Geometry: see drawing. Coordinates: mm, zero at the bounding-box minimum. A direction names the side the tool comes from. Coordinates: 2 decimals unless noted, no trailing zeros. Write each loop counter-clockwise with the first axis right and the second up, starting at its lowest first coordinate (ties: lowest second). Pieces come first, ordered by that corner, then holes. Notation, with made-up numbers: M 6,66.25 L 55,66.25 A17 ccw 55,84.25 Z; hole C 71,65.25 d10. An arc over 180 degrees is marked long. Answer as CSV lines item,"result". Start each with the question number.
1. Section C-C on x = 5. Return the cut outline in (y, z).
2. Section A-A on x = 14. Return the cut outline in (y, z), plus the area to 3 significant figures.
3. Contact query for flat-ended pins moving along their axis: pin 1 Ø5 at (y, z) = (6, 6.5) entering from -X; pin 2 Ø3.5 at (x, z) = (35, 18.5) entering from +Y; pin 3 Ø5.5 at (x, y) = (14.5, 9) entering from +Z; pin 4 Ø3.5 at (x, z) = (5, 18.5) entering from -Y. Output: stop coordinate, or through.
4. Section B-B on y = 3.5. Return the cut outline in (x, z).
5. Mould query, pull axis X, two halves, no side actions, for the marked faces 6, 7, 8 and 9. Classes: pulls with the +X half, pulls with the -X half, needs draft (parallel to the pull), parting line crosses it, or undercut.
6. Section D-D on y = 18. Return the cut outline in (x, z), plus the area to 3 significant figures.
7. Reachability of the marked faces 1, 2, 3, 4 and 5 from +Z, -Z, +X, -X, +Y, -Y: full face, straight path, thin tool, end or side. Return the list, or none.
8. Line query: probe 1 along Y at (x, z) = (14.1, 6.5); probe 2 along X at (y, z) = (14, 2.75); probe 3 along Y at (x, z) = (23, 5.5). Output: solid intervals per line, ascending. Write a range as [from, to].
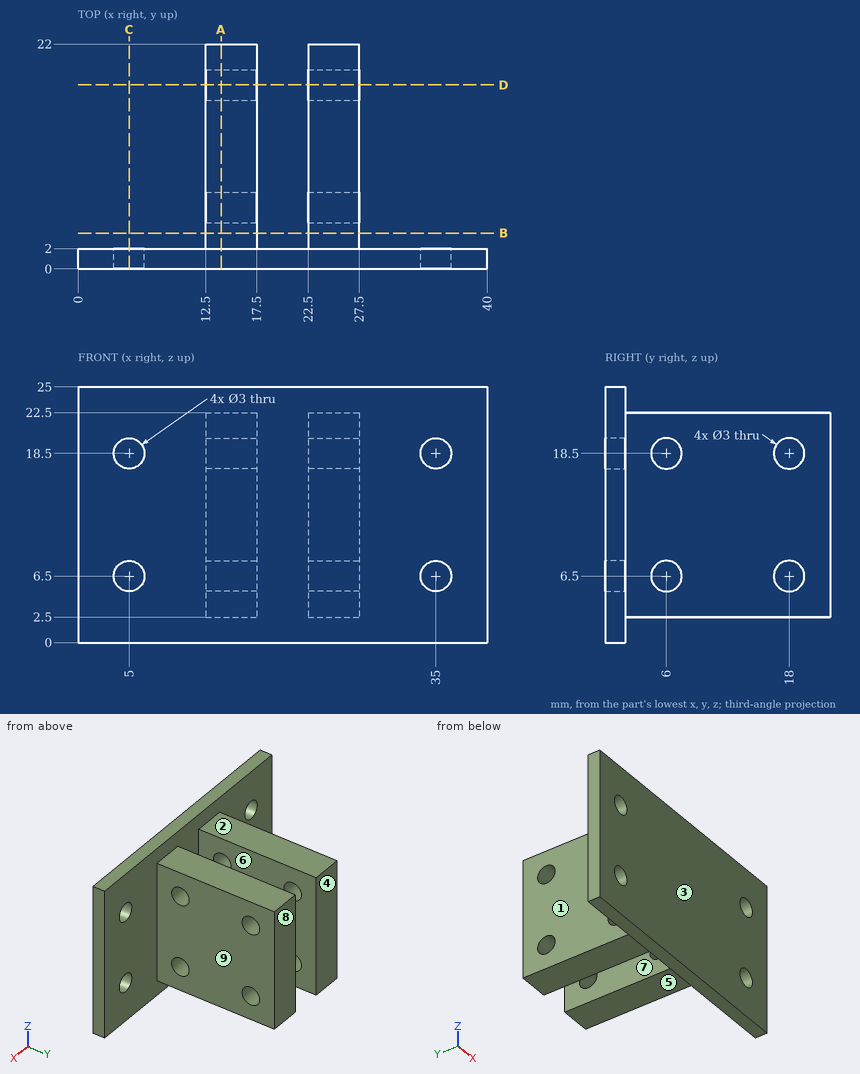
Values:
1,outline,"M 0,0 L 2,0 L 2,5 L 0,5 Z; M 0,8 L 2,8 L 2,17 L 0,17 Z; M 0,20 L 2,20 L 2,25 L 0,25 Z"
2,outline,"M 0,0 L 2,0 L 2,2.5 L 22,2.5 L 22,22.5 L 2,22.5 L 2,25 L 0,25 Z; hole C 6,6.5 d3; hole C 6,18.5 d3; hole C 18,6.5 d3; hole C 18,18.5 d3"
2,area,"422 mm²"
3,pin 1,"x = 12.5"
3,pin 2,"y = 2"
3,pin 3,"z = 22.5"
3,pin 4,"y = 0"
4,outline,"M 12.5,2.5 L 17.5,2.5 L 17.5,22.5 L 12.5,22.5 Z; M 22.5,2.5 L 27.5,2.5 L 27.5,22.5 L 22.5,22.5 Z"
5,face 6,"undercut"
5,face 7,"undercut"
5,face 8,"needs draft"
5,face 9,"pulls with the +X half"
6,outline,"M 12.5,2.5 L 17.5,2.5 L 17.5,5 L 12.5,5 Z; M 12.5,8 L 17.5,8 L 17.5,17 L 12.5,17 Z; M 12.5,20 L 17.5,20 L 17.5,22.5 L 12.5,22.5 Z; M 22.5,2.5 L 27.5,2.5 L 27.5,5 L 22.5,5 Z; M 22.5,8 L 27.5,8 L 27.5,17 L 22.5,17 Z; M 22.5,20 L 27.5,20 L 27.5,22.5 L 22.5,22.5 Z"
6,area,"140 mm²"
7,face 1,"+Z, -Z, -X, +Y"
7,face 2,"+Z, +X, -X, +Y"
7,face 3,"+Z, -Z, +X, -X, -Y"
7,face 4,"+Z, -Z, +X, -X, +Y"
7,face 5,"-Z, +X, -X, +Y"
8,probe 1,"[0, 4.5], [7.5, 16.5], [19.5, 22]"
8,probe 2,"[12.5, 17.5], [22.5, 27.5]"
8,probe 3,"[0, 4.88], [7.12, 16.88], [19.12, 22]"
